Autodesk Inventor part; units mm, degrees
ref_plane "YZ Plane" through (0, 0, 0) normal (1, 0, 0) x (0, 1, 0)
ref_plane "XZ Plane" through (0, 0, 0) normal (0, 1, 0) x (-1, 0, 0)
ref_plane "XY Plane" through (0, 0, 0) normal (0, 0, 1) x (1, 0, 0)
sketch "スケッチ1" plane through (0, 0, 0) normal (0, 0, 1) x (1, 0, 0)
  line L0 (475, -31) -> (-475, -31)
  line L1 (-475, -31) -> (-475, 31)
  line L2 (-475, 31) -> (475, 31)
  line L3 (475, 31) -> (475, -31)
  line L4 (475, -31) -> (-475, 31) construction
  line L5 (-475, -31) -> (475, 31) construction
  point P0 (0, 0)
  dimension "d0" = 62
  dimension "d1" = 950
extrude "プレート1" add sketch "スケッチ1" along normal blind 1.5
sketch "スケッチ2" plane through (475, -32.5, 3) normal (0, -1, 0) x (1, 0, 0)
  line L0 (-950, 0) -> (0, 0)
  line L1 (0, 0) -> (0, 72)
  line L2 (0, 72) -> (-950, 72)
  line L3 (-950, 72) -> (-950, 0)
edge flange "フランジ1" height 75 angle 90 thickness 1.5 bend radius 1.5 thickness toward (0, -1, 0) relief tear relief width 1.5 relief depth 0.75 edges at (0, -31, 1.5) wall of the first edge with corners at (-475, -32.5, 3) (475, -32.5, 3) (475, -32.5, 75) (-475, -32.5, 75)
bend "曲げ1"
corner "コーナー1"
sketch "スケッチ3" plane through (475, -31, 76.5) normal (0, 0, 1) x (1, 0, 0)
  line L0 (-950, 0) -> (0, 0)
  line L1 (0, 0) -> (0, 7)
  line L2 (0, 7) -> (-950, 7)
  line L3 (-950, 7) -> (-950, 0)
edge flange "フランジ2" height 10 angle 90 thickness 1.5 bend radius 1.5 thickness toward (0, 0, 1) relief tear relief width 1.5 relief depth 0.75 edges at (0, -32.5, 75) wall of the first edge with corners at (-475, -31, 76.5) (475, -31, 76.5) (475, -24, 76.5) (-475, -24, 76.5)
bend "曲げ2"
corner "コーナー2"
sketch "スケッチ4" plane through (0, 0, 1.5) normal (0, 0, 1) x (1, 0, 0)
  line L0 (-475, -31) -> (-475, 31)
  line L1 (475, -31) -> (-475, -31)
  line L2 (475, 31) -> (475, -31)
  line L3 (-475, 31) -> (475, 31)
  line L4 (-465, 21) -> (465, 21)
  point P0 (0, 0)
  point P1 (-232.5, 21)
  point P2 (0, 21)
  point P3 (232.5, 21)
  dimension "d23" = 10
  dimension "d24" = 10
  dimension "d25" = 10
  dimension "d26" = 930
  dimension "d27" = 232.5
  dimension "d28" = 232.5
  dimension "d29" = 232.5
hole "穴1" at (-465, 21, 1.5) at (-232.5, 21, 1.5) at (0, 21, 1.5) at (232.5, 21, 1.5) at (465, 21, 1.5) direction (0, 0, -1) diameter 5.3 end through all
sketch "スケッチ5" plane through (-475, -32.5, 3) normal (0, 1, 0) x (1, 0, 0)
  line L0 (950, 0) -> (0, 0)
  line L1 (0, -72) -> (0, 0)
  line L2 (0, -72) -> (950, -72)
  line L3 (950, -72) -> (950, 0)
  line L4 (930, -54) -> (930, -39)
  line L5 (0, 1.5) -> (950, 1.5)
  line L6 (930, -54) -> (910, -54)
  line L7 (910, -54) -> (910, -39)
  line L8 (910, -39) -> (930, -39)
  line L9 (930, -39) -> (930, -54)
  point P0 (475, 3)
  point P1 (930, -46.5)
  dimension "d37" = 15
  dimension "d38" = 48
  dimension "d39" = 20
  dimension "d40" = 20
hole "穴2" at (455, -32.5, 57) at (455, -32.5, 42) at (435, -32.5, 57) at (435, -32.5, 42) direction (0, -1, 0) diameter 3.242 end through all
mirror "ミラー1" about plane through (0, 0, 0) normal (1, 0, 0) of "穴2"
fillet "フィレット1" radius 2 4 edges at (-475, 31, 0.75) (-475, -24, 77.25) (475, 31, 0.75) (475, -24, 77.25)
equation "\"d35\" = Thickness"
equation "\"d2\" = Thickness"
equation "\"d3\" = BendReliefWidth"
equation "\"d4\" = BendReliefDepth"
equation "\"d5\" = MinimumRemnant"
equation "\"d6\" = TransitionRadius"
equation "\"d9\" = BendRadius"
equation "\"d10\" = CornerReliefSize"
equation "\"d11\" = GapSize"
equation "\"d12\" = JacobiRadiusSize"
equation "\"d13\" = BendReliefWidth"
equation "\"d14\" = BendReliefDepth"
equation "\"d15\" = MinimumRemnant"
equation "\"d16\" = TransitionRadius"
equation "\"d19\" = BendRadius"
equation "\"d20\" = CornerReliefSize"
equation "\"d21\" = GapSize"
equation "\"d22\" = JacobiRadiusSize"
equation "\"BendRadius\" = Thickness"
equation "\"BendReliefWidth\" = Thickness"
equation "\"BendReliefDepth\" = 0.5 * Thickness"
equation "\"CornerReliefSize\" = 4 * Thickness"
equation "\"MinimumRemnant\" = 2 * Thickness"
equation "\"TransitionRadius\" = BendRadius"
equation "\"JacobiRadiusSize\" = BendRadius"
equation "\"GapSize\" = Thickness"
properties part number "DragChain_Guide_A"
Geometry check sheet. Reference: the model listing, model coordinates, mm. Coordinates: 2 decimals unless noted, no trailing zeros. Order: outer loops, then holes, each group sorted by start corner. A loop starts at its lowest first (then second) coordinate and runs counter-clockwise, first axis right, second up. Notation, with made-up numbers: (-36, 38) - (-7, 38) arc R26 ccw to (-7, 76) - close; hole circle Ø9 at (-6, -13.5). An arc over 180 degrees is marked (long way). Answer in a Markdown table with one row per item. Add a question column.
1) Release check for a two-part mould opening along Z. For faces 1 (the flat face through (-475, -33, 42)), 2 (the flat face through (7, -32.5, 38)), 3 (the flat face through (-7, 0, 0)) record: +Z half, -Z half, draft (parallel to the pull), parting line (faces both ways), or undercut.
2) Material ranges on line 1 along X through (y, z) = (21, 0.5); line 2 along Z through (x, y) = (435, -32.95); line 3 along Z through (x, y) = (435, -33.5), recorded low to high. Write a range as [from, to].
3) Cross-section at A-A, the plane x = 391.5. Record the cut outline in (y, z).
4) Gauge pin test, flat ends, axial feed: P1, Ø2, axis at x = -263.5, y = -9.5, coming from the +Z side; P2, Ø5, axis at x = 465, y = 21, coming from the +Z side; P3, Ø0.8, axis at x = 219, z = 77.5, coming from the +Y side. Record the tip position at first contact, or that the pin passes through.
5) Cross-section at B-B, the plane y = 3. Record the cut outline in (x, z), then the cut area to 4 significant figures.
Check result:
| question | item | result |
|---|---|---|
| 1 | face 1 | draft |
| 1 | face 2 | undercut |
| 1 | face 3 | -Z half |
| 2 | line 1 | x = [-475, -467.65], [-462.35, -235.15], [-229.85, -2.65], [2.65, 229.85], [235.15, 462.35], [467.65, 475] |
| 2 | line 2 | z = [0.72, 40.38], [43.62, 55.38], [58.62, 77.28] |
| 2 | line 3 | z = [1.34, 40.38], [43.62, 55.38], [58.62, 76.66] |
| 3 | outline | (-34, 3) arc R3 ccw to (-31, 0) - (31, 0) - (31, 1.5) - (-31, 1.5) arc R1.5 cw to (-32.5, 3) - (-32.5, 75) arc R1.5 cw to (-31, 76.5) - (-24, 76.5) - (-24, 78) - (-31, 78) arc R3 ccw to (-34, 75) - close |
| 4 | P1 | stops at z = 1.5 |
| 4 | P2 | passes through |
| 4 | P3 | stops at y = -24 |
| 5 | outline | (-475, 0) - (475, 0) - (475, 1.5) - (-475, 1.5) - close |
| 5 | area | 1,425 mm² |
